Source: CAD feature listing. Evaluate the final solid. Frame: model axes, mm. A direction names the side the tool comes from. Give positions to 0.01 mm unless a question says otherwise; leave off trailing zeros. Write each loop counter-clockwise with the first axis right and the second up, starting at its lowest first coordinate (ties: lowest second). Pieces come first, ordered by that corner, then holes. Notation, with made-up numbers: (13.25, 70.25) -> (44.25, 70.25) arc R19 cw to (44.25, 87.25) -> close; hole circle Ø4 at (30, -35). An arc over 180 degrees is marked (long way). Write item = value, one per line.
from build123d import *

# Parameters (mm, degrees)
SKETCH1_R           = 43.2
BOSS_EXTRUDE1_DEPTH = 40
SKETCH2_R           = 3
SKETCH2_W           = 20
SKETCH2_H           = 20
CUT_EXTRUDE1_DEPTH  = 50
SKETCH3_W           = 8.5
SKETCH3_H           = 8
SKETCH3_W_2         = 72
SKETCH3_H_2         = 30
CUT_EXTRUDE2_DEPTH  = 27
FILLET1_R           = 5
CUT_EXTRUDE3_START  = -32
SKETCH4_R           = 4
CUT_EXTRUDE3_DEPTH  = 32
SKETCH5_R           = 3.6
CUT_EXTRUDE4_DEPTH  = 4
FILLET3_R           = 5
SKETCH7_R           = 6
CUT_EXTRUDE5_DEPTH  = 36


with BuildPart() as part:
    # Sketch1 → Boss-Extrude1 (new body)
    with BuildSketch(Plane(origin=(0, 0, 0), x_dir=(1, 0, 0), z_dir=(0, 1, 0))):
        Circle(SKETCH1_R)
        with BuildLine():
            Line((0, 43.2), (-65, 43.2))
            Line((-65, 43.2), (-65, 0))
            Line((-65, 0), (-43.2, 0))
            ThreePointArc((-43.2, 0), (-30.547012947, 30.547012947), (0, 43.2))
        make_face()
        with BuildLine():
            Line((65, 43.2), (0, 43.2))
            ThreePointArc((0, 43.2), (30.547012947, 30.547012947), (43.2, 0))
            Line((43.2, 0), (65, 0))
            Line((65, 0), (65, 43.2))
        make_face()
    extrude(amount=BOSS_EXTRUDE1_DEPTH)

    # Sketch2 → Cut-Extrude1 (cut)
    with BuildSketch(Plane(origin=(0, 40, 0), x_dir=(1, 0, 0), z_dir=(0, 1, 0))):
        with Locations(Location((0, 25, 0), (0, 0, 270))):
            Circle(SKETCH2_R)
        with Locations(Location((17.67766953, -17.67766953, 0), (0, 0, 270))):
            Circle(SKETCH2_R)
        with Locations(Location((-17.67766953, -17.67766953, 0), (0, 0, 270))):
            Circle(SKETCH2_R)
        with Locations((48, 25)):
            Rectangle(SKETCH2_W, SKETCH2_H)
        with Locations((-48, 21.6)):
            Rectangle(SKETCH2_W, SKETCH2_H)
    extrude(amount=-CUT_EXTRUDE1_DEPTH, mode=Mode.SUBTRACT)

    # Sketch3 → Cut-Extrude2 (cut)
    with BuildSketch(Plane(origin=(0, 40, 0), x_dir=(1, 0, 0), z_dir=(0, 1, 0))):
        with Locations((4.25, -15.338834765)):
            Rectangle(SKETCH3_W, SKETCH3_H)
        with Locations((-4.25, -15.338834765)):
            Rectangle(SKETCH3_W, SKETCH3_H)
        with Locations((0, 3.661165235)):
            Rectangle(SKETCH3_W_2, SKETCH3_H_2)
    extrude(amount=-CUT_EXTRUDE2_DEPTH, mode=Mode.SUBTRACT)

    # Fillet1
    fillet1_edges = [part.edges().sort_by_distance(p)[0] for p in [
        (-22.25, 13, 11.338834765),
        (22.25, 13, 11.338834765),
        (0, 13, -18.661165235),
    ]]
    fillet(fillet1_edges, radius=FILLET1_R)

    # Sketch4 → Cut-Extrude3 (cut)
    with BuildSketch(Plane(origin=(0, 40, 0), x_dir=(1, 0, 0), z_dir=(0, 1, 0)).offset(CUT_EXTRUDE3_START)):
        with BuildLine():
            Line((43.014416188, 4), (36, 4))
            Line((36, 4), (36, -4))
            Line((36, -4), (43.014416188, -4))
            ThreePointArc((43.014416188, -4), (43.153579106, -2.002151427), (43.2, 0))
            Line((43.2, 0), (47.014416188, 0))
            ThreePointArc((47.014416188, 0), (45.842843313, 2.828427125), (43.014416188, 4))
        make_face()
        with BuildLine():
            Line((36, 4), (23.014416188, 4))
            ThreePointArc((23.014416188, 4), (25.842843313, 2.828427125), (27.014416188, 0))
            ThreePointArc((27.014416188, 0), (25.842843313, -2.828427125), (23.014416188, -4))
            Line((23.014416188, -4), (36, -4))
            Line((36, -4), (36, 4))
        make_face()
        with Locations((23.014416188, 0)):
            Circle(SKETCH4_R)
        with BuildLine():
            ThreePointArc((43.014416188, -4), (45.842843313, -2.828427125), (47.014416188, 0))
            Line((47.014416188, 0), (43.2, 0))
            ThreePointArc((43.2, 0), (43.153579106, -2.002151427), (43.014416188, -4))
        make_face()
    extrude(amount=CUT_EXTRUDE3_DEPTH, mode=Mode.SUBTRACT)

    # Sketch5 → Cut-Extrude4 (cut)
    with BuildSketch(Plane(origin=(0, 40, 0), x_dir=(1, 0, 0), z_dir=(0, 1, 0))):
        with Locations(Location((16, 25.8, 0), (0, 0, 270))):
            Circle(SKETCH5_R)
        with Locations(Location((-16, 25.8, 0), (0, 0, 270))):
            Circle(SKETCH5_R)
        with Locations(Location((0, -28.2, 0), (0, 0, 270))):
            Circle(SKETCH5_R)
    extrude(amount=-CUT_EXTRUDE4_DEPTH, mode=Mode.SUBTRACT)

    # Fillet3
    fillet3_edges = [part.edges().sort_by_distance(p)[0] for p in [
        (-2.002151427, 40, 43.153579106),
        (56.007208094, 40, 0),
        (-54.1, 40, 0),
        (-65, 40, -21.6),
        (65, 40, -21.6),
        (0, 40, -43.2),
    ]]
    fillet(fillet3_edges, radius=FILLET3_R)

    # Sketch7 → Cut-Extrude5 (cut)
    with BuildSketch(Plane(origin=(0, 40, 0), x_dir=(1, 0, 0), z_dir=(0, 1, 0))):
        with Locations(Location((0, 25, 0), (0, 0, 270))):
            Circle(SKETCH7_R)
        with Locations(Location((17.67766953, -17.67766953, 0), (0, 0, 270))):
            Circle(SKETCH7_R)
        with Locations(Location((-17.67766953, -17.67766953, 0), (0, 0, 270))):
            Circle(SKETCH7_R)
    extrude(amount=-CUT_EXTRUDE5_DEPTH, mode=Mode.SUBTRACT)


solid = part.part
(1) Section query A-A (x = 0). Return loops of the section in (y, z), plus the area to 3 significant figures.
Values follow:
outline = (0, -43.2) -> (35, -43.2) arc R5 ccw to (40, -38.2) -> (40, -31) -> (4, -31) -> (4, -28) -> (0, -28) -> close; (0, -22) -> (4, -22) -> (4, -19) -> (40, -19) -> (40, -18.66) -> (18, -18.66) arc R5 cw to (13, -13.66) -> (13, 19.34) -> (40, 19.34) -> (40, 24.6) -> (36, 24.6) -> (36, 31.8) -> (40, 31.8) -> (40, 38.2) arc R5 ccw to (35, 43.2) -> (0, 43.2) -> close
area = 1,940 mm2
(2) Material intervals for line 1 (X direction, y = 12, z = 23); line 2 (Z direction, x = -54.5, y = 24); line 3 (X direction, y = 26, z = -5), sorted ascending.
Values follow:
line_1 = -36.57 to -20.45, -14.91 to 14.91, 20.45 to 36.57
line_2 = -43.2 to -31.6, -11.6 to 0
line_3 = -65 to -36, 36 to 65
(3) Pull-direction query (X, two-part tool) for faces 4 (the face through (1, 17, -43.2)), 5 (the face through (65, 17, -21)), 6 (the face through (-16, 36, -26)), 7 (the face through (-63, 39, -21)); classes: pulls with the +X half, pulls with the -X half, needs draft (parallel to the pull), parting line crosses it, or undercut.
Values follow:
face_4 = needs draft
face_5 = pulls with the +X half
face_6 = undercut
face_7 = pulls with the -X half
(4) Access query for faces 1 (the face through (19.015, 10.465, -0.088)), 2 (the face through (-58, 20, -21)), 3 (the face through (45.87, 23.73, -2.8)). Directions: +Z, -Z, +X, -X, +Y, -Y. A direction counts if a zero-diameter tool reaches every point of the face in a straight line with its end or side. Return the directions, or none.
Values follow:
face_1 = +Y
face_2 = +Y, -Y
face_3 = +Z, +Y
(5) First-contact query: pin 1 (8 mm diameter, centred on x = 14.5, y = 15, fed in from +Z); pin 2 (7 mm diameter, centred on x = -17.68, z = 17.68, fed in from +Y); pin 3 (4 mm diameter, centred on x = 38.5, z = 19, fed in from +Y); pin 4 (12 mm diameter, centred on x = 7.5, z = 7, fed in from +Y). Flat tips, straight axial feed; report the tip coordinate or a pass-through.
Values follow:
pin_1 = 41.9
pin_2 = 4
pin_3 = 39.19
pin_4 = 40
(6) Section query B-B (y = 21). Give the number of separate pieces and of enclosed holes in the cut face, plus the area to 3 significant figures.
Values follow:
separate_pieces = 1
enclosed_holes = 5
area = 5,040 mm2
(7) Section query D-D (y = 10). Return loops of the section in (x, z), plus the area to 3 significant figures.
Values follow:
outline = (-65, -43.2) -> (65, -43.2) -> (65, 0) -> (47.01, 0) arc R4 cw to (43.01, -4) -> (23.01, -4) arc R4 cw to (23.01, 4) -> (43.01, 4) arc R43.2 ccw to (-43.2, 0) -> (-65, 0) -> close; hole (-58, -31.6) -> (-38, -31.6) -> (-38, -11.6) -> (-58, -11.6) -> close; hole circle Ø12 at (-17.68, 17.68); hole circle Ø12 at (0, -25); hole circle Ø12 at (17.68, 17.68); hole (38, -35) -> (58, -35) -> (58, -15) -> (38, -15) -> close
area = 7,210 mm2
